```python
from build123d import *

# Parameters (mm, degrees)
EXTRU_MINCE1_DEPTH           = 3.05
ESQUISSE3_W                  = 5
ESQUISSE3_H                  = 3.328220353
ENL_V_MAT_EXTRU_1_DEPTH      = 10
R_P_TITION_CIRCULAIRE1_COUNT = 2


with BuildPart() as part:
    # Esquisse2 → Extru.-Mince1 (new body, symmetric)
    with BuildSketch(Plane.XY):
        with BuildLine():
            Line((0.867691044, -3.516497462), (1.284684178, -2.477324095))
            ThreePointArc((1.284684178, -2.477324095), (1.304066655, -2.262192987), (1.201715788, -2.071978966))
            Line((1.201715788, -2.071978966), (0.211890589, -1.082153766))
            ThreePointArc((0.211890589, -1.082153766), (0.05506857, -0.847453029), (0, -0.570604633))
            Line((0, -0.570604633), (0, 0))
            Line((0, 0), (2.05, 0))
            ThreePointArc((2.05, 0), (2.580330086, 0.219669914), (2.8, 0.75))
            Line((2.8, 0.75), (2.8, 1.400152821))
            ThreePointArc((2.8, 1.400152821), (2.702061046, 1.892525191), (2.423154503, 2.309938332))
            Line((2.423154503, 2.309938332), (1.63248823, 3.100604604))
            ThreePointArc((1.63248823, 3.100604604), (1.418134189, 3.618101038), (1.63248823, 4.135597473))
            Line((1.63248823, 4.135597473), (1.979898987, 4.48300823))
            ThreePointArc((1.979898987, 4.48300823), (2.787260417, 6.196112604), (2.31953586, 8.031267314))
            ThreePointArc((2.31953586, 8.031267314), (2.164350637, 8.664278157), (2.458268281, 9.245997676))
            Line((2.458268281, 9.245997676), (2.8, 9.563603836))
            Line((2.8, 9.563603836), (3.004233324, 9.343856824))
            Line((3.004233324, 9.343856824), (2.662501605, 9.026250664))
            ThreePointArc((2.662501605, 9.026250664), (2.462413038, 8.630236925), (2.568057559, 8.199305896))
            ThreePointArc((2.568057559, 8.199305896), (3.085895462, 6.167527467), (2.192031022, 4.270876196))
            Line((2.192031022, 4.270876196), (1.844620265, 3.923465439))
            ThreePointArc((1.844620265, 3.923465439), (1.718134189, 3.618101038), (1.844620265, 3.312736638))
            Line((1.844620265, 3.312736638), (2.635286537, 2.522070366))
            ThreePointArc((2.635286537, 2.522070366), (2.979224906, 2.007330221), (3.1, 1.400152821))
            Line((3.1, 1.400152821), (3.1, 0.75))
            ThreePointArc((3.1, 0.75), (2.79246212, 0.00753788), (2.05, -0.3))
            Line((2.05, -0.3), (0.3, -0.3))
            Line((0.3, -0.3), (0.3, -0.570604633))
            ThreePointArc((0.3, -0.570604633), (0.33223243, -0.732648), (0.424022623, -0.870021732))
            Line((0.424022623, -0.870021732), (1.413847823, -1.859846932))
            ThreePointArc((1.413847823, -1.859846932), (1.597973034, -2.202034526), (1.563104716, -2.589046986))
            Line((1.563104716, -2.589046986), (1.146111581, -3.628220353))
            Line((1.146111581, -3.628220353), (0.867691044, -3.516497462))
        make_face()
    extru_mince1 = extrude(amount=EXTRU_MINCE1_DEPTH, both=True)

    # Esquisse3 → Enl_v. mat.-Extru.1 (cut)
    with BuildSketch(Plane(origin=(0, 0, 0), x_dir=(0, 0, -1), z_dir=(1, 0, 0))):
        with Locations((0.55, -1.964110177)):
            Rectangle(ESQUISSE3_W, ESQUISSE3_H)
        with BuildLine():
            Line((3.05, 9.563603836), (1.55, 9.563603836))
            ThreePointArc((1.55, 9.563603836), (2.610660172, 9.124264008), (3.05, 8.063603836))
            Line((3.05, 8.063603836), (3.05, 9.563603836))
        make_face()
        with BuildLine():
            Line((-0.45, 9.563603836), (-3.05, 9.563603836))
            Line((-3.05, 9.563603836), (-3.05, 2.309938332))
            Line((-3.05, 2.309938332), (-1.95, 2.309938332))
            Line((-1.95, 2.309938332), (-1.95, 8.063603836))
            ThreePointArc((-1.95, 8.063603836), (-1.510660172, 9.124264008), (-0.45, 9.563603836))
        make_face()
    enl_v_mat_extru_1 = extrude(amount=ENL_V_MAT_EXTRU_1_DEPTH, mode=Mode.SUBTRACT)

    # R_p_tition circulaire1: Extru.-Mince1, Enl_v. mat.-Extru.1 ×2 about axis
    r_p_tition_circulaire1_axis = Axis((0, 0, 0), (0, 1, 0))
    for i in range(1, R_P_TITION_CIRCULAIRE1_COUNT):
        add(extru_mince1.rotate(r_p_tition_circulaire1_axis, i * 360 / R_P_TITION_CIRCULAIRE1_COUNT))
        add(enl_v_mat_extru_1.rotate(r_p_tition_circulaire1_axis, i * 360 / R_P_TITION_CIRCULAIRE1_COUNT), mode=Mode.SUBTRACT)


solid = part.part
```
Input: part model. Units: mm. Frame: model coordinates. A direction names the side the tool comes from. Coordinates: 2 decimals unless noted, no trailing zeros. Loops run counter-clockwise (first coordinate to the right, second up) from the corner with the lowest first, then second, coordinate; pieces in that order, holes last.
Q1. Set-up query: faces 4 (the flat face through (-0.71, -1.58, -2.51)), 5 (the cylindrical face through (2.785, 6.169, -0.515)), 6 (the cylindrical face through (-2.976, 2.015, -0.043)). Return all of +Z, -Z, +X, -X, +Y, -Y with unobstructed straight access to the full face (end or side cutting, diameter ignored); none if empty.
Results are:
face 4: +Z, -Z, +X
face 5: +Z, -Z
face 6: +Z, -Z, -X
Q2. Line query: line 1 along Y through (x, z) = (1.25, 2.25); line 2 along Y through (x, z) = (-2, 1); line 3 along Y through (x, z) = (-1, -1). Output: solid intervals per line, ascending.
Results are:
line 1: y = -3.37 to -2.56, -2.13 to -1.7, -0.3 to 0
line 2: y = -0.3 to 0, 2.73 to 3.16, 4.08 to 4.5
line 3: y = -0.3 to 0
Q3. Section A-A, the plane y = 8.5. Return the cut outline in (x, z), and give its area (3 significant figures).
Results are:
outline: (-2.46, -1.89) - (-2.16, -1.89) - (-2.16, 2.99) - (-2.46, 2.99) - close; (2.16, -2.99) - (2.46, -2.99) - (2.46, 1.89) - (2.16, 1.89) - close
area: 2.93 mm2
Q4. Mould query, pull axis Y, two halves, no side actions, for faces 1 (the cylindrical face through (-2.48, 9.06, -1.57)), 2 (the flat face through (0, 0, 0)), 3 (the flat face through (-1.36, -3.1, -2.51)). Classes: +Y half, -Y half, draft (parallel to the pull), parting line (faces both ways), or undercut.
Results are:
face 1: +Y half
face 2: undercut
face 3: -Y half
Q5. Contact query for flat-ended pins moving along their axis: pin 1 (2 mm diameter, centred on x = -1.5, z = 2.5, fed in from +Y); pin 2 (1.8 mm diameter, centred on x = -1, y = -2.5, fed in from +Z); pin 3 (1 mm diameter, centred on y = 2.5, z = 1, fed in from -X); pin 4 (0.5 mm diameter, centred on x = 0.5, y = -2.5, fed in from -Z). Output: stop coordinate, or through.
Results are:
pin 1: stops at y = 9.28
pin 2: stops at z = -1.95
pin 3: stops at x = -2.98
pin 4: passes through
